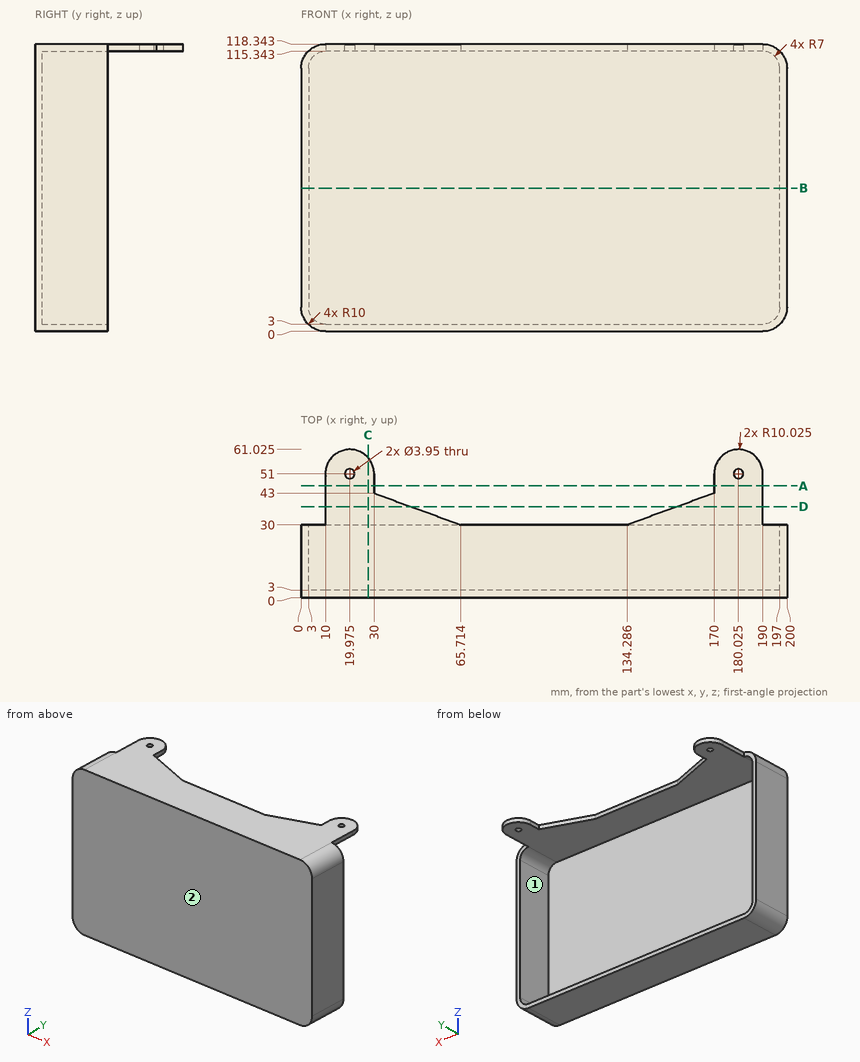
The drawing under review shows one solid part. Ordinate dimensions are in mm from its lowest x, y, z. A direction names the side the tool comes from. Round coordinates to 2 decimals unless told otherwise and drop trailing zeros. Loops run counter-clockwise (first coordinate to the right, second up) from the corner with the lowest first, then second, coordinate; pieces in that order, holes last. Notation, with made-up numbers: (-14, 73.5) - (2, 73.5) arc R25 cw to (2, 103.5) - close; hole circle Ø8 at (-2.75, 52.5). An arc over 180 degrees is marked (long way). Use a Markdown table: item, result. Add a question column.
Q1. Add section D-D (y = 37.5). State the section outline as (x, z) points, plus the area to 3 significant figures.
Q2. Insertion check: pin 1 Ø3.5 at (y, z) = (36, 116.5) entering from -X; pin 2 Ø6 at (x, z) = (69.5, 74) entering from +Y; pin 3 Ø3.5 at (x, y) = (180.025, 51) entering from -Z; pin 4 Ø1.5 at (y, z) = (37, 116.5) entering from +X. Each pin has a flat end and moves straight along its axis. Give the tip position at first contact, or say it passes through.
Q3. For probe 1 along Z at (x, y) = (75, 29.5); probe 2 along X at (y, z) = (18.5, 89.5); probe 3 along Z at (x, y) = (39, 34.5), list the stretches that pass through material, from the lowest coordinate up.
Q4. Add section A-A (y = 46). State the section outline as (x, z) points, plus the area to 3 significant figures.
Q5. Add section C-C (x = 27.5). State the section outline as (y, z) points.
Q6. Machinability: for the marked faces 1 and 2, which of the approach directions +Z, -Z, +X, -X, +Y, -Y give a long, thin tool a straight path to every point of the face, cutting with its end or side? Answer none if there is none.
Q7. Add section B-B (z = 59). State the section outline as (x, y) points.
Worked answers:
| question | item | result |
|---|---|---|
| 1 | outline | (10, 115.34) - (45.11, 115.34) - (45.11, 118.34) - (10, 118.34) - close; (154.89, 115.34) - (190, 115.34) - (190, 118.34) - (154.89, 118.34) - close |
| 1 | area | 211 mm² |
| 2 | pin 1 | x = 10 |
| 2 | pin 2 | y = 3 |
| 2 | pin 3 | through |
| 2 | pin 4 | x = 190 |
| 3 | probe 1 | 0 to 3, 115.34 to 118.34 |
| 3 | probe 2 | 0 to 3, 197 to 200 |
| 3 | probe 3 | 115.34 to 118.34 |
| 4 | outline | (10, 115.34) - (30, 115.34) - (30, 118.34) - (10, 118.34) - close; (170, 115.34) - (190, 115.34) - (190, 118.34) - (170, 118.34) - close |
| 4 | area | 120 mm² |
| 5 | outline | (0, 0) - (30, 0) - (30, 3) - (3, 3) - (3, 115.34) - (57.62, 115.34) - (57.62, 118.34) - (0, 118.34) - close |
| 6 | face 1 | +Y |
| 6 | face 2 | +Z, -Z, +X, -X, -Y |
| 7 | outline | (0, 0) - (200, 0) - (200, 30) - (197, 30) - (197, 3) - (3, 3) - (3, 30) - (0, 30) - close |
